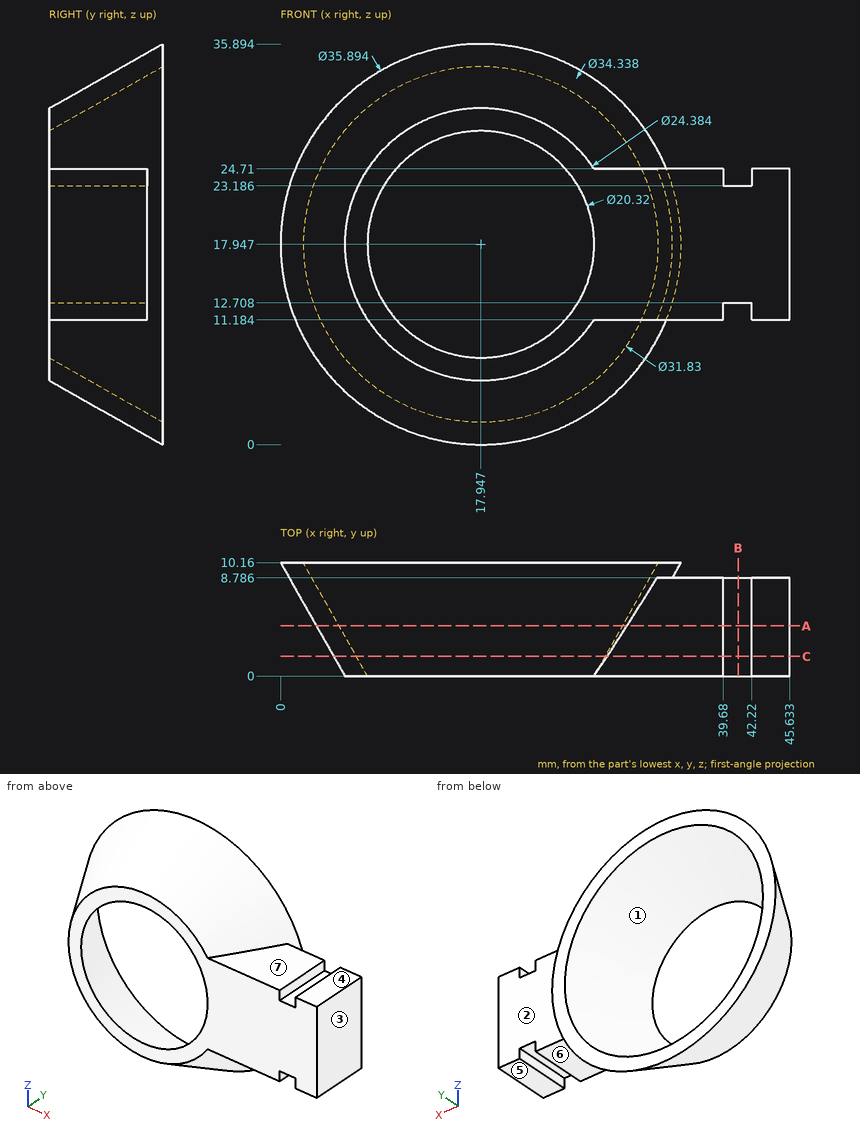
Source: three-view drawing plus pictorial views. Frame: mm from the lowest corner of the part. A direction names the side the tool comes from. Round coordinates to 2 decimals unless told otherwise and drop trailing zeros. Order: outer loops, then holes, each group sorted by start corner. A loop starts at its lowest first (then second) coordinate and runs counter-clockwise, first axis right, second up. Notation, with made-up numbers: (44, -28) - (69, -28) arc R18 cw to (69, -6) - close; hole circle Ø10 at (74, -1). An arc over 180 degrees is marked (long way). Use a Markdown table: item, result.
1. Section A-A on y = 4.5. Return the cut outline in (x, z) (1 decimal).
Evaluation:
| item | result |
|---|---|
| outline | (31, 11.2) - (39.7, 11.2) - (39.7, 12.7) - (42.2, 12.7) - (42.2, 11.2) - (45.6, 11.2) - (45.6, 24.7) - (42.2, 24.7) - (42.2, 23.2) - (39.7, 23.2) - (39.7, 24.7) - (31, 24.7) arc R14.7 ccw (long way) to start; hole circle Ø25.4 at (17.9, 17.9) |
2. Section B-B on x = 41. Return the cut outline in (y, z) (1 decimal).
Evaluation:
| item | result |
|---|---|
| outline | (0, 12.7) - (8.8, 12.7) - (8.8, 23.2) - (0, 23.2) - close |
3. Mould query, pull axis X, two halves, no side actions, for the marked faces 1, 2 and 3. Classes: +X half, -X half, draft (parallel to the pull), parting line (faces both ways), or undercut.
Evaluation:
| item | result |
|---|---|
| face 1 | undercut |
| face 2 | draft |
| face 3 | +X half |
4. Access query for the marked faces 4, 5, 6 and 7. Directions: +Z, -Z, +X, -X, +Y, -Y. A direction counts if a zero-diameter tool reaches every point of the face in a straight line with its end or side. Return the directions, or none.
Evaluation:
| item | result |
|---|---|
| face 4 | +Z, +X, +Y, -Y |
| face 5 | -Z, +X, +Y, -Y |
| face 6 | -Z, +X, -Y |
| face 7 | +Z, +X, -Y |
5. Section C-C on y = 1.75. Return the cut outline in (x, z) (1 decimal), then the cut area to 3 significant figures.
Evaluation:
| item | result |
|---|---|
| outline | (29.3, 11.2) - (39.7, 11.2) - (39.7, 12.7) - (42.2, 12.7) - (42.2, 11.2) - (45.6, 11.2) - (45.6, 24.7) - (42.2, 24.7) - (42.2, 23.2) - (39.7, 23.2) - (39.7, 24.7) - (29.3, 24.7) arc R13.2 ccw (long way) to start; hole circle Ø22.3 at (17.9, 17.9) |
| area | 352 mm^2 |
6. First-contact query: pin 1 (1.3 mm diameter, centred on x = 40.5, y = 3.5, fed in from +Z); pin 2 (2 mm diameter, centred on x = 20.5, z = 29, fed in from +Y) (1 decimal); pin 3 (0.8 mm diameter, centred on y = 5, z = 24, fed in from -X) (1 decimal). Flat tips, straight axial feed; report the tip coordinate or a pass-through.
Evaluation:
| item | result |
|---|---|
| pin 1 | z = 23.19 |
| pin 2 | y = 3.9 |
| pin 3 | x = 3.9 |
7. Material intervals for probe 1 along X at (y, z) = (2, 24) (1 decimal); probe 2 along Z at (x, y) = (36, 2.5) (1 decimal); probe 3 along Z at (x, y) = (25, 6.25) (1 decimal), sorted ascending.
Evaluation:
| item | result |
|---|---|
| probe 1 | 6.1 to 8.4, 27.5 to 39.7, 42.2 to 45.6 |
| probe 2 | 11.2 to 24.7 |
| probe 3 | 3.9 to 6.2, 29.7 to 32 |
